```python
from build123d import *

# Parameters (mm, degrees)
SKETCH1_W             = 6.9
SKETCH1_H             = 20
BOSS_EXTRUDE1_DEPTH   = 1
SKETCH4_R             = 1.9
BOSS_EXTRUDE2_DEPTH   = 0.8
M3X0_5_TAPPED_HOLE1_D = 2.5


with BuildPart() as part:
    # Sketch1 → Boss-Extrude1 (new body)
    with BuildSketch(Plane(origin=(0, 0, 0), x_dir=(1, 0, 0), z_dir=(0, 1, 0))):
        Rectangle(SKETCH1_W, SKETCH1_H)
    extrude(amount=BOSS_EXTRUDE1_DEPTH)

    # Sketch4 → Boss-Extrude2 (add)
    with BuildSketch(Plane.XZ):
        with Locations((0, -7)):
            Circle(SKETCH4_R)
    boss_extrude2 = extrude(amount=BOSS_EXTRUDE2_DEPTH)

    # Mirror2: Boss-Extrude2 across plane
    add(boss_extrude2.mirror(Plane.XY))

    # M3x0.5 Tapped Hole1 (through all)
    with Locations(Plane(origin=(0, 1, 0), x_dir=(1, 0, 0), z_dir=(0, 1, 0))):
        with Locations((0, 7)):
            m3x0_5_tapped_hole1 = Hole(M3X0_5_TAPPED_HOLE1_D / 2)

    # Mirror1: M3x0.5 Tapped Hole1 across plane
    add(m3x0_5_tapped_hole1.mirror(Plane.XY), mode=Mode.SUBTRACT)


solid = part.part
```
Could you check a few things on this model? Use its own coordinates, in mm. A direction names the side the tool comes from. Coordinates: 2 decimals unless noted, no trailing zeros. Write each loop counter-clockwise with the first axis right and the second up, starting at its lowest first coordinate (ties: lowest second). Pieces come first, ordered by that corner, then holes. Notation, with made-up numbers: (-38.75, 34.25) -> (-13.75, 34.25) arc R25 ccw to (-13.75, 55.25) -> close; hole circle Ø1 at (-21.75, -35). An arc over 180 degrees is marked (long way). Return JSON: item names as keys, results as strings.
(1) Imagine slicing it at D-D, the plane y = 0.4. Please give me the cut outline in (x, z).
Numbers:
{"outline": "(-3.45, -10) -> (3.45, -10) -> (3.45, 10) -> (-3.45, 10) -> close; hole circle Ø2.5 at (0, -7); hole circle Ø2.5 at (0, 7)"}
(2) Imagine slicing it at C-C, the plane y = -0.55. Please give me the cut outline in (x, z), then the cut area to 3 significant figures.
Numbers:
{"outline": "circle Ø3.8 at (0, -7); circle Ø3.8 at (0, 7); hole circle Ø2.5 at (0, -7); hole circle Ø2.5 at (0, 7)", "area": "12.9 mm2"}
(3) I need wall thicknesses on L1, parallel to Z at x = 0, y = 0.6; L2, parallel to X at y = 0.3, z = -7; L3, parallel to X at y = -0.25, z = 7. Which ranges of each line are inside material? Lowest first, please.
Numbers:
{"L1": "z = -10 to -8.25, -5.75 to 5.75, 8.25 to 10", "L2": "x = -3.45 to -1.25, 1.25 to 3.45", "L3": "x = -1.9 to -1.25, 1.25 to 1.9"}
(4) Which directions (+Z, -Z, +X, -X, +Y, -Y) give clear straight access to the entire face, cutting with the end or side of a thin tool? Please do faces 4 (the flat face through (0, 0.5, -10)), 5 (the cylindrical face through (-0.247, -0.394, 5.116)).
Numbers:
{"face 4": "-Z, +X, -X, +Y, -Y", "face 5": "-Y"}
(5) I'm going to push a flat-ended pin straight in: pin 1 (1.5 mm diameter, centred on x = 0, z = -7, fed in from +Y). Where does the tip first touch, or does it pass through?
Numbers:
{"pin 1": "passes through"}
(6) We'd pull the mould along Z, two halves only. Please class faces 1 (the flat face through (-3.45, 0.5, 0.1)), 2 (the flat face through (0, 0.5, 10)), 3 (the cylindrical face through (-0.247, -0.394, -5.116)): +Z half, -Z half, draft (parallel to the pull), parting line (faces both ways), or undercut.
Numbers:
{"face 1": "draft", "face 2": "+Z half", "face 3": "undercut"}
(7) Imagine slicing it at A-A, the plane z = 7. Please give me the cut outline in (x, y), then the cut area to 3 significant figures.
Numbers:
{"outline": "(-3.45, 0) -> (-1.9, 0) -> (-1.9, -0.8) -> (-1.25, -0.8) -> (-1.25, 1) -> (-3.45, 1) -> close; (1.25, -0.8) -> (1.9, -0.8) -> (1.9, 0) -> (3.45, 0) -> (3.45, 1) -> (1.25, 1) -> close", "area": "5.44 mm2"}
(8) Imagine slicing it at B-B, the plane x = 0. Please give me the cut outline in (y, z).
Numbers:
{"outline": "(-0.8, -8.9) -> (0, -8.9) -> (0, -10) -> (1, -10) -> (1, -8.25) -> (-0.8, -8.25) -> close; (-0.8, -5.75) -> (1, -5.75) -> (1, 5.75) -> (-0.8, 5.75) -> (-0.8, 5.1) -> (0, 5.1) -> (0, -5.1) -> (-0.8, -5.1) -> close; (-0.8, 8.25) -> (1, 8.25) -> (1, 10) -> (0, 10) -> (0, 8.9) -> (-0.8, 8.9) -> close"}
